Part print with two shaded views. Sizes in mm from the minimum x, y, z corner. Round coordinates to 2 decimals unless told otherwise and drop trailing zeros. Order: outer loops, then holes, each group sorted by start corner. A loop starts at its lowest first (then second) coordinate and runs counter-clockwise, first axis right, second up. Notation, with made-up numbers: (59.25, 8) - (85.25, 8) arc R22 ccw to (85.25, 32) - close; hole circle Ø7 at (80.25, 3.5). An arc over 180 degrees is marked (long way). Use one line per item in the form item = value.
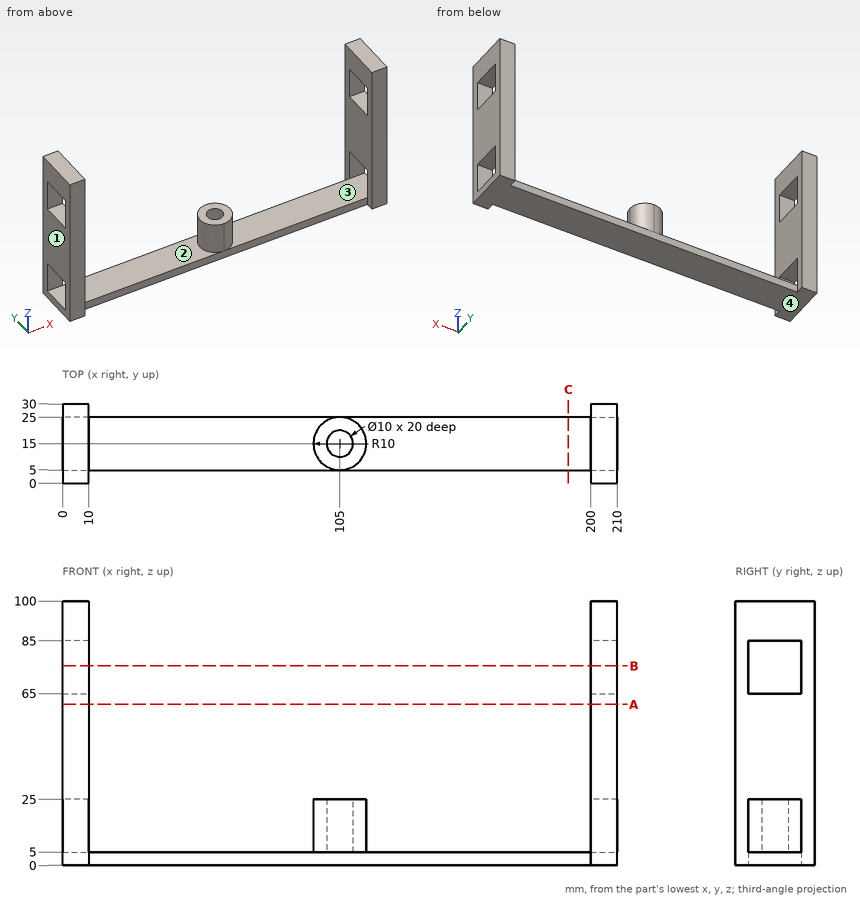
(1) Probe probe 1 along X at (y, z) = (2, 88); probe 2 along Y at (x, z) = (105, 19.75); probe 3 along Z at (x, y) = (53, 11.5). List the from-to ranges inside material, lowest first. Write a range as [from, to].
Report:
probe_1 = [0, 10], [200, 210]
probe_2 = [5, 10], [20, 25]
probe_3 = [0, 5]
(2) Slice it at C-C on x = 191.5. Give the cut face in (y, z).
Report:
outline = (5, 0) - (25, 0) - (25, 5) - (5, 5) - close
(3) Slice it at A-A on z = 61. Give the cut face in (x, y).
Report:
outline = (0, 0) - (10, 0) - (10, 30) - (0, 30) - close; (200, 0) - (210, 0) - (210, 30) - (200, 30) - close
(4) Slice it at B-B on z = 75.5. Give the cut face in (x, y).
Report:
outline = (0, 0) - (10, 0) - (10, 5) - (0, 5) - close; (0, 25) - (10, 25) - (10, 30) - (0, 30) - close; (200, 0) - (210, 0) - (210, 5) - (200, 5) - close; (200, 25) - (210, 25) - (210, 30) - (200, 30) - close
(5) Pull direction Z, two halves, no side cores. Call the marked faces 1, 2, 3 and 4: released by +Z, released by -Z, zero draft, split by the parting line, or undercut.
Report:
face_1 = zero draft
face_2 = undercut
face_3 = undercut
face_4 = released by -Z
(6) Pin check, flat tips, straight feed: pin 1 (8 mm diameter, centred on x = 203.5, y = 10.5, fed in from -Z); pin 2 (1 mm diameter, centred on x = 83.5, y = 7, fed in from +Z); pin 3 (5.5 mm diameter, centred on x = 115.5, z = 2.5, fed in from +Y); pin 4 (8 mm diameter, centred on x = 103, y = 14, fed in from +Z). Stop position of each tip, or through.
Report:
pin_1 = 0
pin_2 = 5
pin_3 = 25
pin_4 = 25
